For this review, take the finished solid that the model builds, in its own axes (mm). Round coordinates to 2 decimals unless told otherwise and drop trailing zeros. Write each loop counter-clockwise with the first axis right and the second up, starting at its lowest first coordinate (ties: lowest second). Pieces come first, ordered by that corner, then holes.
Autodesk Inventor part; units mm, degrees
ref_plane "YZ Plane" through (0, 0, 0) normal (1, 0, 0) x (0, 1, 0)
ref_plane "XZ Plane" through (0, 0, 0) normal (0, 1, 0) x (-1, 0, 0)
ref_plane "XY Plane" through (0, 0, 0) normal (0, 0, 1) x (1, 0, 0)
sketch "Szkic1" plane through (0, 0, 0) normal (0, 1, 0) x (-1, 0, 0)
  line L0 (4, 30) -> (-4, 30)
  line L1 (-4, 30) -> (-4, -30)
  line L2 (-4, -30) -> (4, -30)
  line L3 (4, -30) -> (4, 30)
  point P0 (0, 0)
  point P1 (4, 0)
  point P2 (0, -30)
  dimension "d0" = 8
  dimension "d1" = 60
extrude "Wyciągnięcie proste1" add sketch "Szkic1" along normal blind 5
sketch "Szkic2" plane through (0, 5, 0) normal (0, 1, 0) x (1, 0, 0)
  circle A0 centre (0, 0) radius 0.5
  dimension "d4" = 1
extrude "Wyciągnięcie proste2" cut sketch "Szkic2" against normal blind 2.5
properties part number "Smiglo"
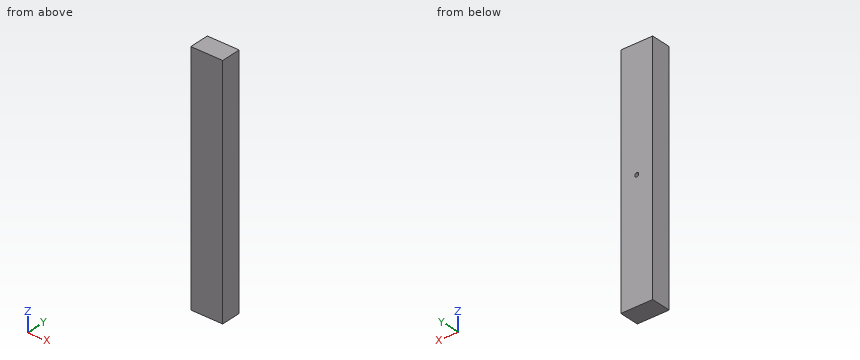
(1) We need section A-A, the plane z = 0. Give the boundary of the cut face in (x, y).
Geometry check:
outline: (-4, 0) - (4, 0) - (4, 5) - (0.5, 5) - (0.5, 2.5) - (-0.5, 2.5) - (-0.5, 5) - (-4, 5) - close
(2) For pin 1 Ø3 at (x, z) = (-1, -20.5) entering from -Y; pin 2 Ø0.8 at (x, z) = (0, 0) entering from +Y, all flat-tipped, find the tip position at first contact; note any pin that passes through.
Geometry check:
pin 1: stops at y = 0
pin 2: stops at y = 2.5
(3) For line 1 along Z through (x, y) = (0, 3.4); line 2 along X through (y, z) = (3.55, 0), list the stretches that pass through material, from the lowest coordinate up.
Geometry check:
line 1: z = -30 to -0.5, 0.5 to 30
line 2: x = -4 to -0.5, 0.5 to 4
